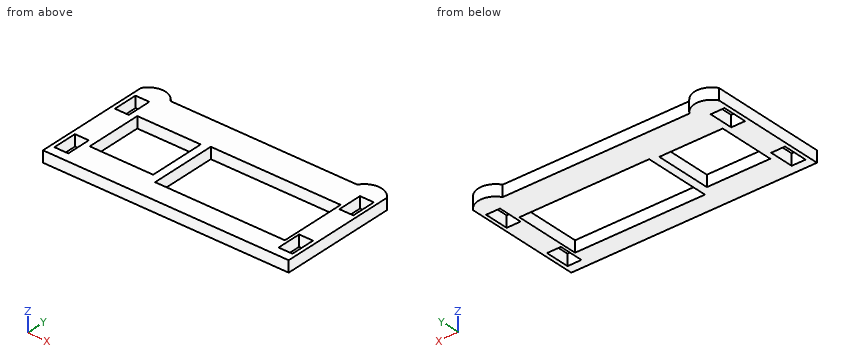
from build123d import *

# Parameters (mm, degrees)
F0_W     = 3.7
F0_H     = 6.53
F0_W_2   = 16.9
F0_H_2   = 15.12
F0_W_3   = 34.6
F0_H_3   = 17.7038
F1_DEPTH = 3


with BuildPart() as f1:
    # F0 (on Top) → F1 (new body)
    with BuildSketch(Plane.XY):
        with BuildLine():
            Line((-28.684194, 9.618534), (-28.684194, -21.551466))
            Line((-28.684194, -21.551466), (36.795806, -21.551466))
            Line((36.795806, -21.551466), (36.795806, 9.618534))
            ThreePointArc((36.795806, 9.618534), (32.870806, 11.798534), (28.945806, 9.618534))
            Line((28.945806, 9.618534), (-20.834194, 9.618534))
            ThreePointArc((-20.834194, 9.618534), (-24.759194, 11.798534), (-28.684194, 9.618534))
        make_face()
        with Locations((-25.818194, -15.876466)):
            Rectangle(F0_W, F0_H, mode=Mode.SUBTRACT)
        with Locations((-13.904194, -6.691466)):
            Rectangle(F0_W_2, F0_H_2, mode=Mode.SUBTRACT)
        with Locations((33.929806, -15.876466)):
            Rectangle(F0_W, F0_H, mode=Mode.SUBTRACT)
        with Locations((13.995806, -7.340166)):
            Rectangle(F0_W_3, F0_H_3, mode=Mode.SUBTRACT)
        with Locations((-25.818194, 3.353534)):
            Rectangle(F0_W, F0_H, mode=Mode.SUBTRACT)
        with Locations((34.022406, 3.353534)):
            Rectangle(F0_W, F0_H, mode=Mode.SUBTRACT)
    extrude(amount=F1_DEPTH)


solid = f1.part
Model file for the job. Use its own axes, mm. Give positions to 0.01 mm unless a question says otherwise; leave off trailing zeros. Order: outer loops, then holes, each group sorted by start corner. A loop starts at its lowest first (then second) coordinate and runs counter-clockwise, first axis right, second up. Notation, with made-up numbers: (61.25, 43) - (87.25, 43) arc R22 ccw to (87.25, 62) - close; hole circle Ø10 at (38.25, 31.5). An arc over 180 degrees is marked (long way). One line per item, written item: value.
Item 1: Slice it at C-C (z = 1.3). Give the number of separate pieces and of enclosed holes in the cut face, then the cut area to 3 significant figures.
Response values:
separate pieces: 1
enclosed holes: 6
area: 1,100 mm2
Item 2: Slice it at B-B (x = 19). List the corners of the cut face in (y, z).
Response values:
outline: (-21.55, 0) - (-16.19, 0) - (-16.19, 3) - (-21.55, 3) - close; (1.51, 0) - (9.62, 0) - (9.62, 3) - (1.51, 3) - close
Item 3: Pin check, flat tip, straight feed: pin 1 Ø0.9 at (x, z) = (-11, 1.5) entering from +Y. Stop position of the tip, or through.
Response values:
pin 1: y = 9.62
Item 4: Slice it at D-D (y = -15.5). List the corners of the cut face in (x, z), then the cut area to 3 significant figures.
Response values:
outline: (-28.68, 0) - (-27.67, 0) - (-27.67, 3) - (-28.68, 3) - close; (-23.97, 0) - (-3.3, 0) - (-3.3, 3) - (-23.97, 3) - close; (31.3, 0) - (32.08, 0) - (32.08, 3) - (31.3, 3) - close; (35.78, 0) - (36.8, 0) - (36.8, 3) - (35.78, 3) - close
area: 70.4 mm2
Item 5: Slice it at A-A (y = 5). List the corners of the cut face in (x, z).
Response values:
outline: (-28.68, 0) - (-27.67, 0) - (-27.67, 3) - (-28.68, 3) - close; (-23.97, 0) - (32.17, 0) - (32.17, 3) - (-23.97, 3) - close; (35.87, 0) - (36.8, 0) - (36.8, 3) - (35.87, 3) - close
Item 6: Wall check: line 1 (X direction, y = 2.5, z = 0.3); line 2 (X direction, y = -11.5, z = 1.55); line 3 (X direction, y = 1, z = 2). Give the ranges that are in metal, low to high.
Response values:
line 1: -28.68 to -27.67, -23.97 to 32.17, 35.87 to 36.8
line 2: -28.68 to -22.35, -5.45 to -3.3, 31.3 to 36.8
line 3: -28.68 to -27.67, -23.97 to -3.3, 31.3 to 32.17, 35.87 to 36.8
